Could you check a few things on this model? Use its own coordinates, in mm. Face numbers are marked on the shaded views. A direction names the side the tool comes from. Coordinates: 2 decimals unless noted, no trailing zeros. Write each loop counter-clockwise with the first axis right and the second up, starting at its lowest first coordinate (ties: lowest second). Pieces come first, ordered by that corner, then holes. Notation, with made-up numbers: (20, 67.5) - (41, 67.5) arc R31 ccw to (41, 104.5) - close; hole circle Ø10 at (67, -4.5). An arc over 180 degrees is marked (long way). Write item = value, one per line. Start each with the question number.
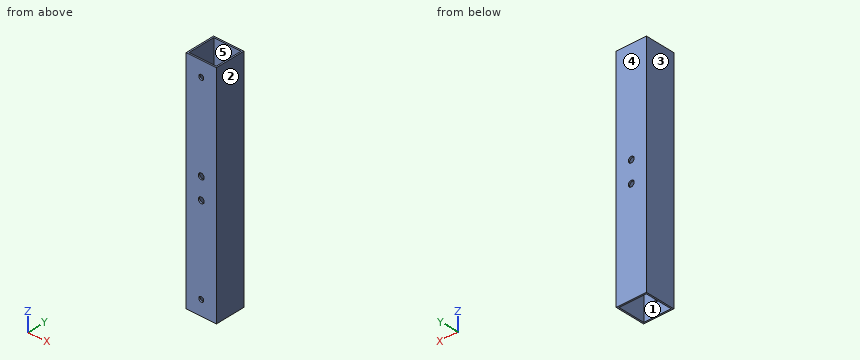
```python
from build123d import *

# Parameters (mm, degrees)
SKETCH_1_W          = 20
SKETCH_1_H          = 20
SKETCH_1_W_2        = 18
SKETCH_1_H_2        = 18
EXTRUDE_1_DEPTH     = 150
SKETCH_3_R          = 1.95
CUT_EXTRUDE_2_DEPTH = 153.643375225
CUT_EXTRUDE_3_REACH = 154.643
SKETCH_4_R          = 1.65


with BuildPart() as part:
    # 草图1 → 拉伸-薄壁1 (new body)
    with BuildSketch(Plane.XY):
        with Locations((10, -10)):
            Rectangle(SKETCH_1_W, SKETCH_1_H)
        with Locations((10, -10)):
            Rectangle(SKETCH_1_W_2, SKETCH_1_H_2, mode=Mode.SUBTRACT)
    extrude(amount=EXTRUDE_1_DEPTH)

    # 草图3 → 切除-拉伸2 (cut, through all)
    with BuildSketch(Plane.XZ.offset(20)):
        with Locations(Location((10, 82, 0), (0, 0, 270))):
            Circle(SKETCH_3_R)
        with Locations(Location((10, 68, 0), (0, 0, 270))):
            Circle(SKETCH_3_R)
    extrude(amount=-CUT_EXTRUDE_2_DEPTH, mode=Mode.SUBTRACT)

    # 草图4 → 切除-拉伸3 (cut, up to next)
    with BuildSketch(Plane.XZ.offset(20), mode=Mode.PRIVATE) as cut_extrude_3_sk1:
        with Locations(Location((10, 140, 0), (0, 0, 270))):
            Circle(SKETCH_4_R)
    cut_extrude_3_tool1 = extrude(cut_extrude_3_sk1.sketch, amount=-CUT_EXTRUDE_3_REACH, mode=Mode.PRIVATE) & part.part
    # 草图4 → 切除-拉伸3 (cut, up to next)
    with BuildSketch(Plane.XZ.offset(20), mode=Mode.PRIVATE) as cut_extrude_3_sk2:
        with Locations(Location((10, 10, 0), (0, 0, 270))):
            Circle(SKETCH_4_R)
    cut_extrude_3_tool2 = extrude(cut_extrude_3_sk2.sketch, amount=-CUT_EXTRUDE_3_REACH, mode=Mode.PRIVATE) & part.part
    add(cut_extrude_3_tool1.solids().sort_by_distance((10, -20, 140))[0], mode=Mode.SUBTRACT)
    add(cut_extrude_3_tool2.solids().sort_by_distance((10, -20, 10))[0], mode=Mode.SUBTRACT)


solid = part.part
```
1) Suppose I cut it at D-D on x = 10. State how many separate pieces and enclosed holes the cut face has, plus the area to 3 significant figures.
2) If I drill on probe 1 along Y at (x, z) = (13.75, 88.5); probe 2 along X at (y, z) = (-8.25, 93.5); probe 3 along X at (y, z) = (-19.5, 10), over which ranges is the centre line in solid material (lowest first)? Write a range as [from, to].
3) Suppose I cut it at B-B on x = 15.75. Please give me the cut outline in (y, z).
4) Suppose I cut it at A-A on z = 82. Please give me the cut outline in (x, y), plus the area to 3 significant figures.
5) Thinking about a two-plate mould opening in X: for the marked faces 1, 2 and 3, which applies, +X half, -X half, draft (parallel to the pull), parting line (faces both ways), or undercut?
6) Which directions (+Z, -Z, +X, -X, +Y, -Y) give clear straight access to the entire face, cutting with the end or side of a thin tool? Please do the marked faces 4 and 5.
7) Suppose I cut it at C-C on y = -11.5. Please give me the cut outline in (x, z).
8) For P1, Ø3, axis at x = 10, z = 68, coming from the +Y side, with a flat end and sliding along its axis, tell me the tip position at first contact or that it passes through.
Reply:
q1.separate_pieces = 8
q1.enclosed_holes = 0
q1.area = 278 mm^2
q2.probe_1 = [-20, -19], [-1, 0]
q2.probe_2 = [0, 1], [19, 20]
q2.probe_3 = [0, 8.35], [11.65, 20]
q3.outline = (-20, 0) - (-19, 0) - (-19, 150) - (-20, 150) - close; (-1, 0) - (0, 0) - (0, 150) - (-1, 150) - close
q4.outline = (0, -20) - (8.05, -20) - (8.05, -19) - (1, -19) - (1, -1) - (8.05, -1) - (8.05, 0) - (0, 0) - close; (11.95, -20) - (20, -20) - (20, 0) - (11.95, 0) - (11.95, -1) - (19, -1) - (19, -19) - (11.95, -19) - close
q4.area = 68.2 mm^2
q5.face_1 = undercut
q5.face_2 = +X half
q5.face_3 = -X half
q6.face_4 = +Z, -Z, +X, -X, +Y
q6.face_5 = +Z, -Z
q7.outline = (0, 0) - (1, 0) - (1, 150) - (0, 150) - close; (19, 0) - (20, 0) - (20, 150) - (19, 150) - close
q8.P1 = through
